Build history of the part. All positions in model axes, mm. Face numbers are marked on the shaded views. A direction names the side the tool comes from. Round coordinates to 2 decimals unless told otherwise and drop trailing zeros. Loops run counter-clockwise (first coordinate to the right, second up) from the corner with the lowest first, then second, coordinate; pieces in that order, holes last. Notation, with made-up numbers: (54, -30.75) - (63, -30.75) arc R15 ccw to (63, -10.75) - close; hole circle Ø4 at (3, 62). An arc over 180 degrees is marked (long way). Use one line per item in the form item = value. Start each with the question number.
Q1. 3-axis set-ups, long thin cutter, end or side, ignore diameter. For the marked faces 1 and 2: which of +Z, -Z, +X, -X, +Y, -Y reach the whole face in a straight line?
Q2. Saw through at B-B (x = -11). Give the cut face in (y, z).
Q3. Saw through at C-C (y = 54). Give the cut face in (x, z).
Q4. Drill centre lines: line 1 (X direction, y = 44.5, z = 11.5); line 2 (Y direction, x = -7.5, z = 12.5). Where is each one in solid material? Low to high.
Q5. Saw through at A-A (z = 15). Give the cut face in (x, y).
Q6. Mould opens along Y. For the marked faces 3, 4 and 5 say: released by +Y, released by -Y, zero draft, split by the parting line, or undercut.
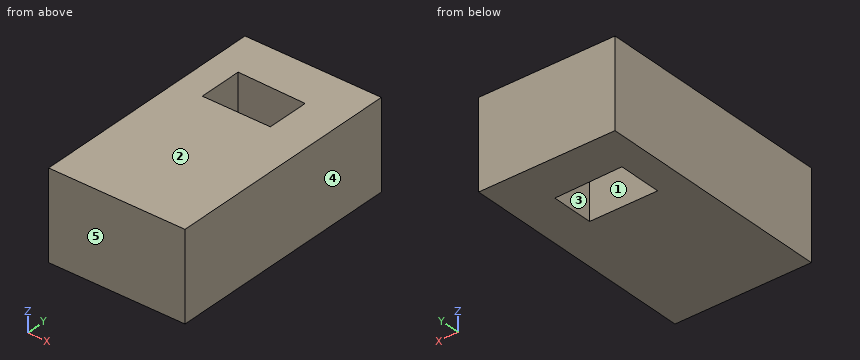
```python
from build123d import *

# Parameters (mm, degrees)
F0_W     = 19.7146944702
F0_H     = 44.4659888744
F0_W_2   = 8.1341895928
F1_DEPTH = 25.4


with BuildPart() as f1:
    # F0 (on Top) → F1 (new body)
    with BuildSketch(Plane.XY):
        Polygon((11.6561325267, 0), (11.6561325267, 56.5538331866), (0, 44.4659888744), (0, 0), align=None)
        Polygon((0, 44.4659888744), (11.6561325267, 56.5538331866), (0, 56.7677064351), align=None)
        Polygon((0, 56.7677064351), (11.6561325267, 56.5538331866), (11.6561325267, 69.5050880313), (0, 69.5050880313), align=None)
        with Locations((-9.8573472351, 22.2329944372)):
            Rectangle(F0_W, F0_H)
        Polygon((-19.7146944702, 57.1294426918), (0, 56.7677064351), (0, 69.5050880313), (-27.848884063, 69.5050880313), (-27.848884063, 44.4659888744), align=None)
        Polygon((-19.7146944702, 44.4659888744), (-19.7146944702, 57.1294426918), (-27.848884063, 44.4659888744), align=None)
        with Locations((-23.7817892666, 22.2329944372)):
            Rectangle(F0_W_2, F0_H)
    extrude(amount=F1_DEPTH)


solid = f1.part
```
Report:
q1.face_1 = +Z, -Z
q1.face_2 = +Z, +X, -X, +Y, -Y
q2.outline = (0, 0) - (44.47, 0) - (44.47, 25.4) - (0, 25.4) - close; (56.97, 0) - (69.51, 0) - (69.51, 25.4) - (56.97, 25.4) - close
q3.outline = (-27.85, 0) - (-19.71, 0) - (-19.71, 25.4) - (-27.85, 25.4) - close; (0, 0) - (11.66, 0) - (11.66, 25.4) - (0, 25.4) - close
q4.line_1 = -27.85 to -19.71, 0 to 11.66
q4.line_2 = 0 to 44.47, 56.91 to 69.51
q5.outline = (-27.85, 0) - (11.66, 0) - (11.66, 69.51) - (-27.85, 69.51) - close; hole (-19.71, 44.47) - (0, 44.47) - (0, 56.77) - (-19.71, 57.13) - close
q6.face_3 = undercut
q6.face_4 = zero draft
q6.face_5 = released by -Y
